Drawing for the job (mm, zero at the part's lowest x, y, z). Give positions to 0.01 mm unless a question says otherwise; leave off trailing zeros. Order: outer loops, then holes, each group sorted by start corner. A loop starts at its lowest first (then second) coordinate and runs counter-clockwise, first axis right, second up. Notation, with made-up numbers: (50, 83.25) - (80, 83.25) arc R13 cw to (80, 93.25) - close; hole circle Ø11 at (-5.75, 28.5). An arc over 180 degrees is marked (long way). Use a Markdown table: item, result.
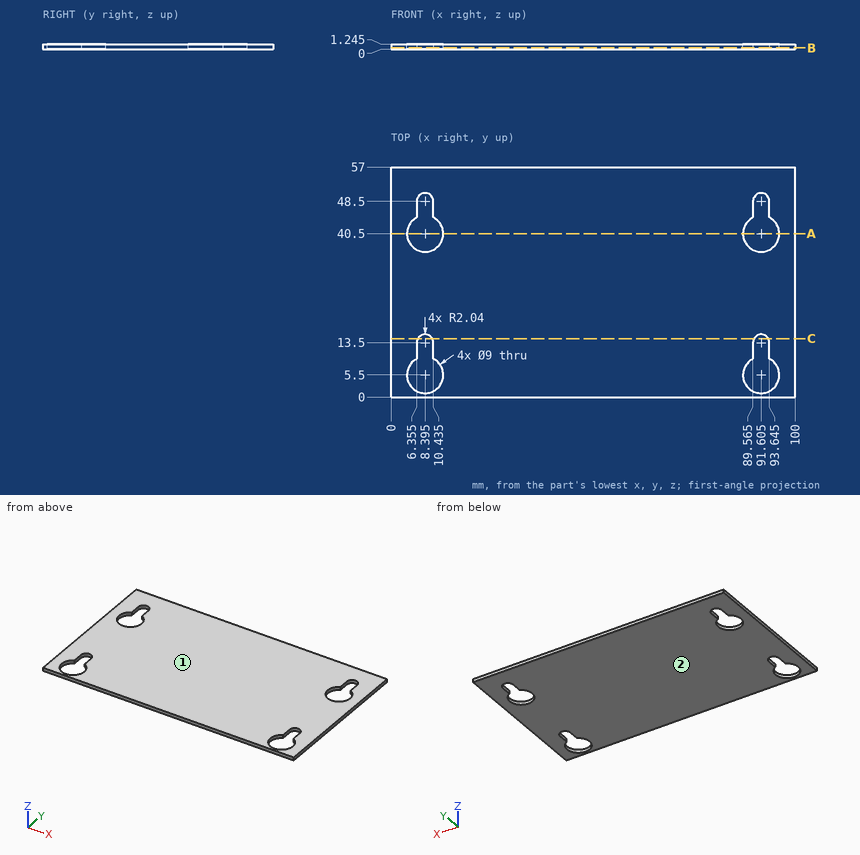
1) Slice it at C-C (y = 14.5). Write the cut outline in (x, z) (3 decimals).
Computed:
| item | result |
|---|---|
| outline | (0, 0) - (6.617, 0) - (6.617, 1.245) - (0, 1.245) - close; (10.173, 0) - (89.827, 0) - (89.827, 1.245) - (10.173, 1.245) - close; (93.383, 0) - (100, 0) - (100, 1.245) - (93.383, 1.245) - close |
2) Two-plate mould, pull along Z, no slides. Class the marked faces 1 and 2: +Z half, -Z half, draft (parallel to the pull), parting line (faces both ways), or undercut.
Computed:
| item | result |
|---|---|
| face 1 | +Z half |
| face 2 | -Z half |
3) Slice it at B-B (z = 0.3). Write the cut outline in (x, y) (3 decimals), and give its area (3 significant figures).
Computed:
| item | result |
|---|---|
| outline | (0, 0) - (100, 0) - (100, 57) - (0, 57) - close; hole (6.355, 9.511) arc R4.5 ccw (long way) to (10.435, 9.511) - (10.435, 13.5) arc R2.04 ccw to (6.355, 13.5) - close; hole (6.355, 44.511) arc R4.5 ccw (long way) to (10.435, 44.511) - (10.435, 48.5) arc R2.04 ccw to (6.355, 48.5) - close; hole (89.565, 9.511) arc R4.5 ccw (long way) to (93.645, 9.511) - (93.645, 13.5) arc R2.04 ccw to (89.565, 13.5) - close; hole (89.565, 44.511) arc R4.5 ccw (long way) to (93.645, 44.511) - (93.645, 48.5) arc R2.04 ccw to (89.565, 48.5) - close |
| area | 5,360 mm² |
4) Pin check, flat tip, straight feed: P1, Ø5.5, axis at x = 91.605, y = 40.5, coming from the +Z side. Stop position of the tip, or through.
Computed:
| item | result |
|---|---|
| P1 | passes through |
5) Wall check: line 1 (X direction, y = 5.5, z = 0.85) (3 decimals); line 2 (X direction, y = 10.5, z = 0.3) (3 decimals); line 3 (Y direction, x = 5, z = 0.4). Give the ranges that are in metal, low to high. Write a range as from..to.
Computed:
| item | result |
|---|---|
| line 1 | x = 0..3.895, 12.895..87.105, 96.105..100 |
| line 2 | x = 0..6.355, 10.435..89.565, 93.645..100 |
| line 3 | y = 0..2.55, 8.45..37.55, 43.45..57 |
6) Slice it at A-A (y = 40.5). Write the cut outline in (x, z) (3 decimals), and give its area (3 significant figures).
Computed:
| item | result |
|---|---|
| outline | (0, 0) - (3.895, 0) - (3.895, 1.245) - (0, 1.245) - close; (12.895, 0) - (87.105, 0) - (87.105, 1.245) - (12.895, 1.245) - close; (96.105, 0) - (100, 0) - (100, 1.245) - (96.105, 1.245) - close |
| area | 102 mm² |
